Geometry: final body of the model. Coordinates: model frame, mm. Face numbers are marked on the shaded views. A direction names the side the tool comes from. Round coordinates to 2 decimals unless told otherwise and drop trailing zeros. Write each loop counter-clockwise with the first axis right and the second up, starting at its lowest first coordinate (ties: lowest second). Pieces come first, ordered by that corner, then holes. Notation, with made-up numbers: M 56.5,9 L 90.5,9 A18 cw 90.5,27 Z; hole C 40.5,-12.5 d11. An arc over 180 degrees is marked long. Use one line per item in the form item = value. Start each with the question number.
Item 1: Ray query, probe 1 along Y at (x, z) = (44.5, 27.5); probe 2 along X at (y, z) = (23.5, 39); probe 3 along Y at (x, z) = (9, 4). Return the intervals inside material, ascending.
Item 2: Section query D-D (z = 12.5). Return loops of the section in (x, y), and give its area (3 significant figures).
Item 3: Section query C-C (y = 29). Return loops of the section in (x, z).
Item 4: Section query A-A (x = 37.5). Return loops of the section in (y, z), and give its area (3 significant figures).
Item 5: Section query B-B (z = 36.5). Return loops of the section in (x, y).
Item 6: Pin query (flat end, axial travel): pin 1 Ø8 at (y, z) = (13.5, 32.5) entering from -X; pin 2 Ø8.5 at (x, z) = (6, 17.5) entering from -Y; pin 3 Ø7.5 at (y, z) = (29, 29) entering from +X; pin 4 Ø11.5 at (x, z) = (3.5, 34.5) entering from +Y. Return the tip coordinate at first contact, or that it passes through.
Item 7: Reachability of the marked faces 1, 2, 3, 4 and 5 from +Z, -Z, +X, -X, +Y, -Y: full face, straight path, thin tool, end or side. Return the list, or none.
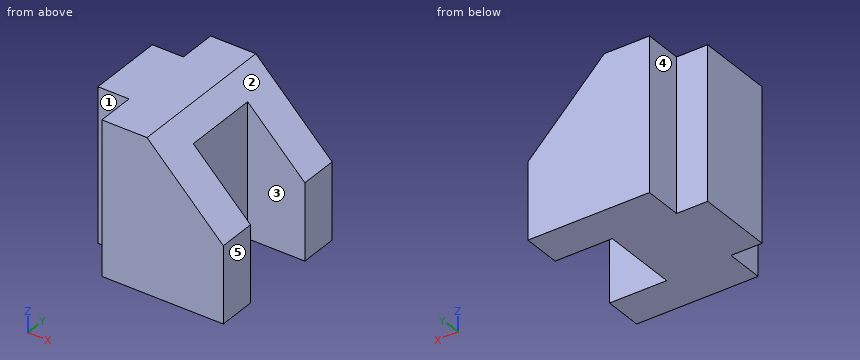
from build123d import *

# Parameters (mm, degrees)
F0_W     = 50.8
F0_H     = 50.8
F1_DEPTH = 50.8
F2_W     = 19.05
F2_H     = 25.4
F3_DEPTH = 50.801
F5_DEPTH = 50.801
F6_W     = 10.347801
F6_H     = 12.7
F7_DEPTH = 50.801


with BuildPart() as f1:
    # F0 (on Top) → F1 (new body)
    with BuildSketch(Plane.XY):
        with Locations((25.4, 25.4)):
            Rectangle(F0_W, F0_H)
    extrude(amount=F1_DEPTH)

    # F2 (on face) → F3 (cut, through all)
    with BuildSketch(Plane.XY.offset(50.8)):
        with Locations((41.275, 25.4)):
            Rectangle(F2_W, F2_H)
    extrude(amount=-F3_DEPTH, mode=Mode.SUBTRACT)

    # F4 (on face) → F5 (cut, through all)
    with BuildSketch(Plane.XZ):
        Polygon((25.4, 50.8), (50.8, 25.4), (50.8, 50.8), align=None)
    extrude(amount=-F5_DEPTH, mode=Mode.SUBTRACT)

    # F6 (on face) → F7 (cut, through all)
    with BuildSketch(Plane.XY.offset(50.8)):
        with Locations((5.1739, 6.35)):
            Rectangle(F6_W, F6_H)
        with Locations((5.1739, 44.45)):
            Rectangle(F6_W, F6_H)
    extrude(amount=-F7_DEPTH, mode=Mode.SUBTRACT)


solid = f1.part
Working result:
q1.probe_1 = 0 to 12.7, 38.1 to 50.8
q1.probe_2 = 0 to 31.75
q1.probe_3 = 12.7 to 38.1
q2.outline = M 0,12.7 L 10.35,12.7 L 10.35,0 L 50.8,0 L 50.8,12.7 L 31.75,12.7 L 31.75,38.1 L 50.8,38.1 L 50.8,50.8 L 10.35,50.8 L 10.35,38.1 L 0,38.1 Z
q2.area = 1,830 mm²
q3.outline = M 0,0 L 31.75,0 L 31.75,44.45 L 25.4,50.8 L 0,50.8 Z
q4.outline = M 0,0 L 12.7,0 L 12.7,38.7 L 0,38.7 Z; M 38.1,0 L 50.8,0 L 50.8,38.7 L 38.1,38.7 Z
q4.area = 983 mm²
q5.outline = M 0,12.7 L 10.35,12.7 L 10.35,0 L 39.7,0 L 39.7,12.7 L 31.75,12.7 L 31.75,38.1 L 39.7,38.1 L 39.7,50.8 L 10.35,50.8 L 10.35,38.1 L 0,38.1 Z
q6.pin_1 = 0
q6.pin_2 = 12.7
q6.pin_3 = 31.75
q6.pin_4 = 38.1
q7.face_1 = +Z, -Z, -X, -Y
q7.face_2 = +Z, +X, +Y, -Y
q7.face_3 = +Z, -Z, +X
q7.face_4 = +Z, -Z, -X, +Y
q7.face_5 = +Z, -Z, +X, +Y, -Y
